Geometry: final body of the model. Coordinates: model frame, mm. A direction names the side the tool comes from. Coordinates: 2 decimals unless noted, no trailing zeros. Loops run counter-clockwise (first coordinate to the right, second up) from the corner with the lowest first, then second, coordinate; pieces in that order, holes last. Notation, with made-up numbers: (41, 85) - (56, 85) arc R18 ccw to (56, 89) - close; hole circle Ø11 at (84, -5). An arc over 180 degrees is marked (long way). Put each result on its own line as item: value. Start each with the question number.
1) Section A-A on z = -16. Output: boundary loops of the cut face in (x, y), and give its area (3 significant figures).
2) Section B-B on y = 32. Output: boundary loops of the cut face in (x, z).
3) Section D-D on y = 43. Output: boundary loops of the cut face in (x, z), and give its area (3 significant figures).
4) Contact query for flat-ended pins moving along their axis: pin 1 Ø14.5 at (x, y) = (30, 28) entering from +Z; pin 2 Ø3.5 at (x, z) = (78.29, -41) entering from +Y; pin 3 Ø1 at (y, z) = (14.5, -16) entering from -X; pin 4 Ø8 at (x, z) = (47, -16) entering from +Y. Output: stop coordinate, or through.
5) Draft query along Z for faces 4 (the flat face through (25, 12, -16)), 5 (the cylindrical face through (45.28, 22.534, -29.747)), 6 (the flat face through (76, 13.925, 14)). Return one class per face: +Z half, -Z half, draft (parallel to the pull), parting line (faces both ways), or undercut.
6) Material intervals for line 1 along Z through (x, y) = (8.5, 14); line 2 along X through (y, z) = (17, -13.5); line 3 along Z through (x, y) = (41, 8.5), sorted ascending. Write a range as from..to.
7) Reachability of faces 1 (the flat face through (65, 15, -16)), 2 (the flat face through (25, 33, 1)), 3 (the cylindrical face through (3, 41, -16)) from +Z, -Z, +X, -X, +Y, -Y: full face, straight path, thin tool, end or side. Return the list, or none.
8) Section C-C on x = 17.5. Output: boundary loops of the cut face in (y, z), and give its area (3 significant figures).
```python
from build123d import *

# Parameters (mm, degrees)
ESQUISSE1_W             = 25
ESQUISSE1_H             = 48
BOSS_EXTRU_1_DEPTH      = 2
ESQUISSE2_R             = 2
BOSS_EXTRU_2_DEPTH      = 32
ESQUISSE3_W             = 25
ESQUISSE3_H             = 48
BOSS_EXTRU_3_DEPTH      = 2
ESQUISSE5_W             = 36
ESQUISSE5_H             = 24
BOSS_EXTRU_4_DEPTH      = 40
ESQUISSE6_R             = 2
ENL_V_MAT_EXTRU_1_DEPTH = 10
ENL_V_MAT_EXTRU_2_DEPTH = 40
ESQUISSE9_W             = 23
ESQUISSE9_H             = 10
BOSS_EXTRU_5_DEPTH      = 23
ESQUISSE10_R            = 2
ENL_V_MAT_EXTRU_3_DEPTH = 23
ESQUISSE11_W            = 23
ESQUISSE11_H            = 10
BOSS_EXTRU_6_DEPTH      = 23
ESQUISSE13_R            = 2
ENL_V_MAT_EXTRU_4_DEPTH = 23
ENL_V_MAT_EXTRU_5_DEPTH = 23
ESQUISSE15_W            = 82
ESQUISSE15_H            = 3.074752109
ESQUISSE15_H_2          = 2.925247891
ENL_V_MAT_EXTRU_6_DEPTH = 10
CONG_1_R                = 1
CONG_2_R                = 1


with BuildPart() as part:
    # Esquisse1 → Boss.-Extru.1 (new body)
    with BuildSketch(Plane.XY):
        with Locations((12.5, 24)):
            Rectangle(ESQUISSE1_W, ESQUISSE1_H)
    extrude(amount=BOSS_EXTRU_1_DEPTH)

    # Esquisse2 → Boss.-Extru.2 (add)
    with BuildSketch(Plane(origin=(0, 0, 0), x_dir=(-1, 0, 0), z_dir=(0, 0, -1))):
        with Locations((-3, 5)):
            Circle(ESQUISSE2_R)
        with Locations((-3, 43)):
            Circle(ESQUISSE2_R)
    extrude(amount=BOSS_EXTRU_2_DEPTH)

    # Esquisse3 → Boss.-Extru.3 (add)
    with BuildSketch(Plane(origin=(0, 0, -32), x_dir=(-1, 0, 0), z_dir=(0, 0, -1))):
        with Locations((-12.5, 24)):
            Rectangle(ESQUISSE3_W, ESQUISSE3_H)
    extrude(amount=BOSS_EXTRU_3_DEPTH)

    # Esquisse5 → Boss.-Extru.4 (add)
    with BuildSketch(Plane(origin=(25, 0, 0), x_dir=(0, 0, -1), z_dir=(1, 0, 0))):
        with Locations((16, 12)):
            Rectangle(ESQUISSE5_W, ESQUISSE5_H)
    extrude(amount=BOSS_EXTRU_4_DEPTH)

    # Esquisse6 → Enlèv. mat.-Extru.1 (cut)
    with BuildSketch(Plane(origin=(65, 0, 0), x_dir=(0, 0, -1), z_dir=(1, 0, 0))):
        with Locations((16, 12)):
            Circle(ESQUISSE6_R)
    extrude(amount=-ENL_V_MAT_EXTRU_1_DEPTH, mode=Mode.SUBTRACT)

    # Esquisse7 → Enlèv. mat.-Extru.2 (cut)
    with BuildSketch(Plane(origin=(65, 0, 0), x_dir=(0, 0, -1), z_dir=(1, 0, 0))):
        with BuildLine():
            Line((8, 24), (8, 33.499215261))
            Line((8, 33.499215261), (-16.874865577, 33.499215261))
            Line((-16.874865577, 33.499215261), (-16.874865577, 0))
            Line((-16.874865577, 0), (8, 0))
            ThreePointArc((8, 0), (-4, 12), (8, 24))
        make_face()
        with BuildLine():
            Line((24, 24), (24, 33.499215261))
            Line((24, 33.499215261), (42.8283548, 33.499215261))
            Line((42.8283548, 33.499215261), (42.8283548, 0))
            Line((42.8283548, 0), (24, 0))
            ThreePointArc((24, 0), (36, 12), (24, 24))
        make_face()
    extrude(amount=-ENL_V_MAT_EXTRU_2_DEPTH, mode=Mode.SUBTRACT)

    # Esquisse9 → Boss.-Extru.5 (add)
    with BuildSketch(Plane.XY.offset(2)):
        with Locations((69.5, 12)):
            Rectangle(ESQUISSE9_W, ESQUISSE9_H)
    extrude(amount=BOSS_EXTRU_5_DEPTH)

    # Esquisse10 → Enlèv. mat.-Extru.3 (cut)
    with BuildSketch(Plane(origin=(0, 17, 0), x_dir=(1, 0, 0), z_dir=(0, 1, 0))):
        with Locations(Location((78.293015344, -21, 0), (0, 0, 270))):
            Circle(ESQUISSE10_R)
        with Locations(Location((78.293015344, -9, 0), (0, 0, 270))):
            Circle(ESQUISSE10_R)
    extrude(amount=-ENL_V_MAT_EXTRU_3_DEPTH, mode=Mode.SUBTRACT)

    # Esquisse11 → Boss.-Extru.6 (add)
    with BuildSketch(Plane(origin=(0, 0, -34), x_dir=(-1, 0, 0), z_dir=(0, 0, -1))):
        with Locations((-69.5, 12)):
            Rectangle(ESQUISSE11_W, ESQUISSE11_H)
    extrude(amount=BOSS_EXTRU_6_DEPTH)

    # Esquisse13 → Enlèv. mat.-Extru.4 (cut)
    with BuildSketch(Plane(origin=(0, 17, 0), x_dir=(1, 0, 0), z_dir=(0, 1, 0))):
        with Locations(Location((78.293015344, 41, 0), (0, 0, 180))):
            Circle(ESQUISSE13_R)
        with Locations(Location((78.293015344, 53, 0), (0, 0, 180))):
            Circle(ESQUISSE13_R)
    extrude(amount=-ENL_V_MAT_EXTRU_4_DEPTH, mode=Mode.SUBTRACT)

    # Esquisse14 → Enlèv. mat.-Extru.5 (cut)
    with BuildSketch(Plane(origin=(0, 17, 0), x_dir=(1, 0, 0), z_dir=(0, 1, 0))):
        Polygon((58, 34), (76, 57), (58, 57), align=None)
        Polygon((58, -2), (76, -25), (58, -25), align=None)
    extrude(amount=-ENL_V_MAT_EXTRU_5_DEPTH, mode=Mode.SUBTRACT)

    # Esquisse15 → Enlèv. mat.-Extru.6 (cut)
    with BuildSketch(Plane(origin=(81, 0, 0), x_dir=(0, 0, -1), z_dir=(1, 0, 0))):
        with Locations((16, 15.462623946)):
            Rectangle(ESQUISSE15_W, ESQUISSE15_H)
        with Locations((16, 8.462623946)):
            Rectangle(ESQUISSE15_W, ESQUISSE15_H_2)
    extrude(amount=-ENL_V_MAT_EXTRU_6_DEPTH, mode=Mode.SUBTRACT)

    # Congé1
    cong_1_edges = [part.edges().sort_by_distance(p)[0] for p in [
        (25, 0, 1),
        (0, 48, 1),
        (25, 48, 1),
        (0, 0, 1),
    ]]
    fillet(cong_1_edges, radius=CONG_1_R)

    # Congé2
    cong_2_edges = [part.edges().sort_by_distance(p)[0] for p in [
        (0, 0, -33),
        (0, 48, -33),
        (25, 48, -33),
        (25, 0, -33),
    ]]
    fillet(cong_2_edges, radius=CONG_2_R)


solid = part.part
```
Answer block:
1. outline: circle Ø4 at (3, 5); circle Ø4 at (3, 43); (25, 0) - (65, 0) - (65, 10) - (55, 10) - (55, 14) - (65, 14) - (65, 24) - (25, 24) - close
1. area: 945 mm²
2. outline: (0, -34) - (25, -34) - (25, -32) - (0, -32) - close; (0, 0) - (25, 0) - (25, 2) - (0, 2) - close
3. outline: (0, -34) - (25, -34) - (25, -32) - (5, -32) - (5, 0) - (25, 0) - (25, 2) - (0, 2) - (0, 0) - (1, 0) - (1, -32) - (0, -32) - close
3. area: 228 mm²
4. pin 1: stops at z = 2
4. pin 2: passes through
4. pin 3: stops at x = 25
4. pin 4: stops at y = 24
5. face 4: undercut
5. face 5: -Z half
5. face 6: draft
6. line 1: z = -34..-32, 0..2
6. line 2: x = 25..65
6. line 3: z = -34..2
7. face 1: +X, +Y, -Y
7. face 2: +Z, +X, +Y
7. face 3: none
8. outline: (0, -34) - (48, -34) - (48, -32) - (0, -32) - close; (0, 0) - (48, 0) - (48, 2) - (0, 2) - close
8. area: 192 mm²
